Input: dimensioned drawing with shaded views. Units: mm. Origin: part minimum x, y, z. A direction names the side the tool comes from. Round coordinates to 2 decimals unless told otherwise and drop trailing zeros. Loops run counter-clockwise (first coordinate to the right, second up) from the corner with the lowest first, then second, coordinate; pieces in that order, holes last. Notation, with made-up numbers: M -11,-30.75 L 6,-30.75 A18 cw 6,-24.75 Z; hole C -4.5,-26.5 d3. An arc over 180 degrees is marked long. Answer as a JSON object with one key per item and string values.
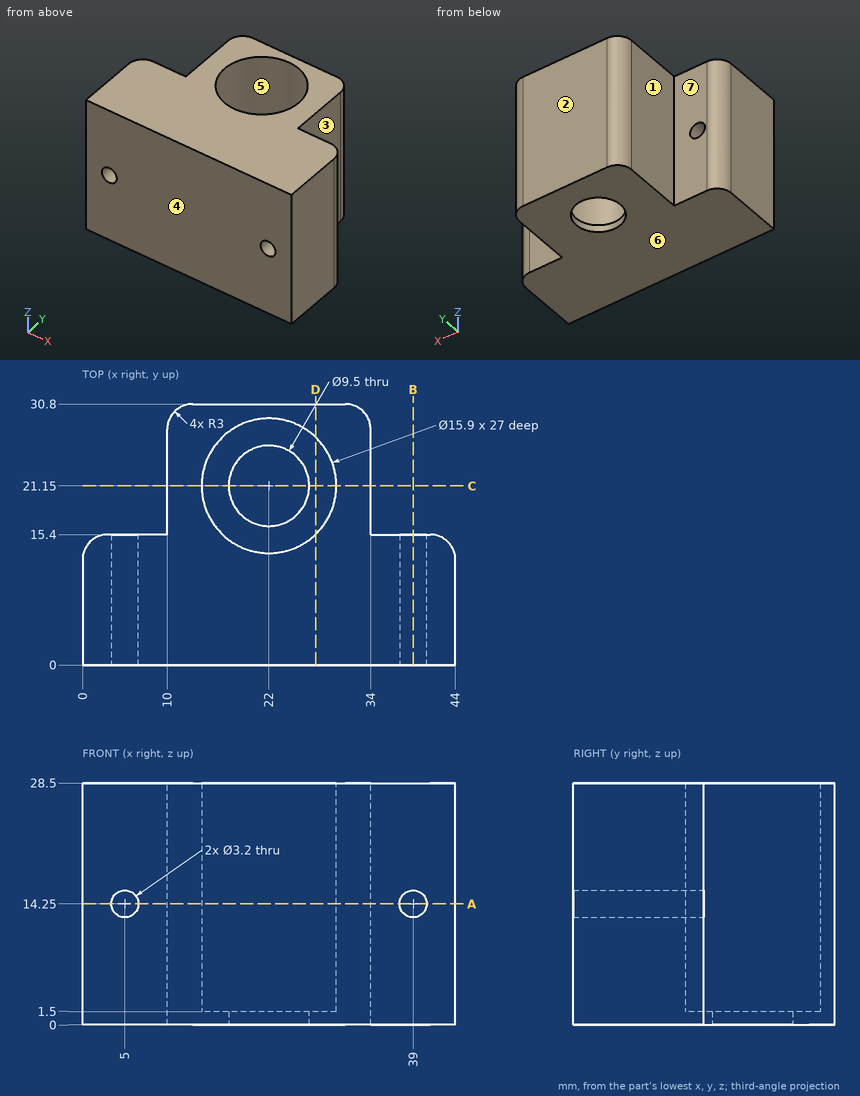
Item 1: Access query for the marked faces 1, 2 and 3. Directions: +Z, -Z, +X, -X, +Y, -Y. A direction counts if a zero-diameter tool reaches every point of the face in a straight line with its end or side. Return the directions, or none.
Answer sheet:
{"face 1": "+Z, -Z, -X, +Y", "face 2": "+Z, -Z, +X, -X, +Y", "face 3": "+Z, -Z, +X, +Y"}
Item 2: Section C-C on y = 21.15. Return the cut outline in (x, z).
Answer sheet:
{"outline": "M 10,0 L 17.25,0 L 17.25,1.5 L 14.05,1.5 L 14.05,28.5 L 10,28.5 Z; M 26.75,0 L 34,0 L 34,28.5 L 29.95,28.5 L 29.95,1.5 L 26.75,1.5 Z"}
Item 3: Section D-D on x = 27.5. Return the cut outline in (y, z).
Answer sheet:
{"outline": "M 0,0 L 30.8,0 L 30.8,28.5 L 26.89,28.5 L 26.89,1.5 L 15.41,1.5 L 15.41,28.5 L 0,28.5 Z"}
Item 4: Section B-B on x = 39. Return the cut outline in (y, z).
Answer sheet:
{"outline": "M 0,0 L 15.4,0 L 15.4,12.65 L 0,12.65 Z; M 0,15.85 L 15.4,15.85 L 15.4,28.5 L 0,28.5 Z"}
Item 5: Contact query for flat-ended pins moving along their axis: pin 1 Ø10 at (y, z) = (20, 10.5) entering from -X; pin 2 Ø11 at (x, y) = (22, 21.15) entering from +Z; pin 3 Ø6 at (y, z) = (19, 18.5) entering from +X. Output: stop coordinate, or through.
Answer sheet:
{"pin 1": "stops at x = 1.5", "pin 2": "stops at z = 1.5", "pin 3": "stops at x = 34"}
Item 6: Section A-A on z = 14.25. Return the cut outline in (x, y).
Answer sheet:
{"outline": "M 0,0 L 3.4,0 L 3.4,15.4 L 3,15.4 A3 ccw 0,12.4 Z; M 6.6,0 L 37.4,0 L 37.4,15.4 L 34,15.4 L 34,27.8 A3 ccw 31,30.8 L 13,30.8 A3 ccw 10,27.8 L 10,15.4 L 6.6,15.4 Z; M 40.6,0 L 44,0 L 44,12.4 A3 ccw 41,15.4 L 40.6,15.4 Z; hole C 22,21.15 d15.9"}
Item 7: Pull-direction query (Y, two-part tool) for the marked faces 4, 5, 6 and 7; classes: pulls with the +Y half, pulls with the -Y half, needs draft (parallel to the pull), parting line crosses it, or undercut.
Answer sheet:
{"face 4": "pulls with the -Y half", "face 5": "undercut", "face 6": "needs draft", "face 7": "pulls with the +Y half"}
Item 8: Line query: probe 1 along Z at (x, y) = (39, 6.25); probe 2 along X at (y, z) = (2, 14.5); probe 3 along Y at (x, z) = (22, 15.25). Output: solid intervals per line, ascending. Write a range as from..to.
Answer sheet:
{"probe 1": "z = 0..12.65, 15.85..28.5", "probe 2": "x = 0..3.42, 6.58..37.42, 40.58..44", "probe 3": "y = 0..13.2, 29.1..30.8"}
